Source: CAD feature listing. Evaluate the final solid. Frame: model axes, mm. A direction names the side the tool comes from. Give positions to 0.01 mm unless a question says otherwise; leave off trailing zeros. Order: outer loops, then holes, each group sorted by start corner. A loop starts at its lowest first (then second) coordinate and runs counter-clockwise, first axis right, second up. Notation, with made-up numbers: M -24.5,65 L 16.5,65 A21 ccw 16.5,103 Z; hole C -1,26 d7. An arc over 180 degrees is marked long. Answer as a JSON object with one key per item and string values. Group by question number.
1. Section query A-A (x = 501). Output: boundary loops of the cut face in (y, z), plus the area to 3 significant figures.
2. Section query C-C (x = 396.5). Output: boundary loops of the cut face in (y, z) (3 decimals), plus the area to 3 significant figures.
3. Pin query (flat end, axial travel): P1, Ø3, axis at x = 348.5, y = 98, coming from the +Z side; P2, Ø3, axis at x = 358.5, z = -241.5, coming from the -Y side; P3, Ø4, axis at y = 49.5, z = -47.5, coming from the -X side; P4, Ø4, axis at y = 26.5, z = -86.5, coming from the -X side. Return the tip coordinate at first contact, or that it passes through.
4. Set-up query: faces 4 (the cylindrical face through (56.771, 74.388, -167.411)), 5 (the flat face through (376, 47, -323.85)). Return all of +Z, -Z, +X, -X, +Y, -Y with unobstructed straight access to the full face (end or side cutting, diameter ignored); none if empty.
5. Material intervals for L1, parallel to Z at x = 387, y = 21.5; L2, parallel to Y at x = 355.5, z = -16, sorted ascending. Write a range as [from, to].
6. Pull-direction query (Z, two-part tool) for faces 1 (the flat face through (376, 50, 0)), 2 (the flat face through (376, 47, -6.35)), 3 (the flat face through (379, 0, -325)); classes: +Z half, -Z half, draft (parallel to the pull), parting line (faces both ways), or undercut.
7. Section query D-D (y = 28). Output: boundary loops of the cut face in (x, z).
8. Section query B-B (z = -49). Output: boundary loops of the cut face in (x, y), plus the area to 3 significant figures.
from build123d import *

# Parameters (mm, degrees)
SKETCH1_W           = 762
SKETCH1_H           = 330.2
BOSS_EXTRUDE1_DEPTH = 101.6
FILLET1_R           = 152.4
SHELL1_T            = -6.35
SKETCH3_W           = 135.128
SKETCH3_H           = 43.18
SKETCH3_W_2         = 50.8
SKETCH3_H_2         = 50.8
CUT_EXTRUDE1_DEPTH  = 127.762


with BuildPart() as part:
    # Sketch1 → Boss-Extrude1 (new body)
    with BuildSketch(Plane(origin=(0, 0, 0), x_dir=(1, 0, 0), z_dir=(0, 1, 0))):
        with Locations((381, 165.1)):
            Rectangle(SKETCH1_W, SKETCH1_H)
    extrude(amount=BOSS_EXTRUDE1_DEPTH)

    # Fillet1
    # the kernel refuses this fillet: 152.4 mm, written as the material it takes off along each edge
    with BuildSketch(Plane(origin=(0, 101.6, -689.410244843), x_dir=(0, -1, 0), z_dir=(0, 0, 1))) as fillet1_piece_1:
        with BuildLine():
            CenterArc((152.4, 143.684097937), FILLET1_R, 180, 70.528779366)
            Line((0, 143.684097937), (-3.048, 143.684097937))
            Line((-3.048, 143.684097937), (-3.048, 0))
            Line((-3.048, 0), (0, -3.048))
            ThreePointArc((0, -3.048), (50.8, -3.048), (100.584, -2.873681959))
            Line((100.584, -2.873681959), (101.6, 0))
        make_face()
    extrude(amount=1048.620489686, mode=Mode.SUBTRACT)

    # Shell1
    shell1_openings = [part.faces().sort_by_distance(p)[0] for p in [
        (381, 0, -165.1),
    ]]
    offset(amount=SHELL1_T, openings=shell1_openings, kind=Kind.INTERSECTION)

    # Sketch3 → Cut-Extrude1 (cut)
    with BuildSketch(Plane(origin=(0, 101.6, 0), x_dir=(1, 0, 0), z_dir=(0, 1, 0))):
        with Locations((339.485069024, 49.525)):
            Rectangle(SKETCH3_W, SKETCH3_H)
        with Locations((649.365069024, 280.675)):
            Rectangle(SKETCH3_W, SKETCH3_H)
        with Locations((649.365069024, 49.525)):
            Rectangle(SKETCH3_W, SKETCH3_H)
        with Locations((339.485069024, 280.675)):
            Rectangle(SKETCH3_W, SKETCH3_H)
        with Locations((494.425069024, 165.1)):
            Rectangle(SKETCH3_W_2, SKETCH3_H_2)
    extrude(amount=-CUT_EXTRUDE1_DEPTH, mode=Mode.SUBTRACT)


solid = part.part
Answer sheet:
{
 "1": {"outline": "M 0,-330.2 L 101.6,-330.2 L 101.6,-190.5 L 95.25,-190.5 L 95.25,-323.85 L 0,-323.85 Z; M 0,-6.35 L 95.25,-6.35 L 95.25,-139.7 L 101.6,-139.7 L 101.6,0 L 0,0 Z", "area": "2,980 mm^2"},
 "2": {"outline": "M 0,-330.2 L 101.6,-330.2 L 101.6,-302.265 L 95.25,-302.265 L 95.25,-323.85 L 0,-323.85 Z; M 0,-6.35 L 95.25,-6.35 L 95.25,-27.935 L 101.6,-27.935 L 101.6,0 L 0,0 Z; M 95.25,-259.085 L 101.6,-259.085 L 101.6,-71.115 L 95.25,-71.115 Z", "area": "2,760 mm^2"},
 "3": {"P1": "z = 0", "P2": "y = 95.25", "P3": "x = 27.22", "P4": "x = 11.19"},
 "4": {"face 4": "+Z, -Z, -X, +Y", "face 5": "-Y"},
 "5": {"L1": "[-330.2, -323.85], [-6.35, 0]", "L2": "[95.25, 101.6]"},
 "6": {"face 1": "+Z half", "face 2": "undercut", "face 3": "draft"},
 "7": {"outline": "M 13.24,-330.2 L 762,-330.2 L 762,0 L 13.24,0 Z; hole M 20.72,-323.85 L 755.65,-323.85 L 755.65,-6.35 L 20.72,-6.35 Z"},
 "8": {"outline": "M 0,0 L 6.75,0 A146.05 cw 143.68,95.25 L 271.92,95.25 L 271.92,101.6 L 143.68,101.6 A152.4 ccw Z; M 407.05,95.25 L 581.8,95.25 L 581.8,101.6 L 407.05,101.6 Z; M 716.93,95.25 L 755.65,95.25 L 755.65,0 L 762,0 L 762,101.6 L 716.93,101.6 Z", "area": "3,970 mm^2"}
}
